For this review, take the finished solid that the model builds, in its own axes (mm). Give positions to 0.01 mm unless a question says otherwise; leave off trailing zeros. Write each loop counter-clockwise with the first axis right and the second up, starting at its lowest first coordinate (ties: lowest second). Pieces come first, ordered by that corner, then holes. Notation, with made-up numbers: M 14.5,-40 L 56.5,-40 A18 cw 56.5,-36 Z; hole C 56,-10 d2. An arc over 180 degrees is marked long. Use one line per item in the form item = value. Start each with the question number.
Q1. For probe 1 along Y at (x, z) = (2, 191); probe 2 along X at (y, z) = (-0.5, -171.5), list the stretches that pass through material, from the lowest coordinate up. Write a range as [from, to].
Q2. Clearance check with flat-ended pins moving along their axes: pin 1 Ø8 at (x, z) = (4.5, -220) entering from +Y; pin 2 Ø2 at (x, z) = (-11.5, -84.5) entering from +Y; pin 3 Ø10 at (x, y) = (11.5, -2) entering from +Z. State where each tip first meets the part, or that it passes through.
Q3. Consider section A-A on z = 134. Write out the cut boundary in (x, y).
```python
from build123d import *

# Parameters (mm, degrees)
SKETCH1_R           = 20
BOSS_EXTRUDE1_DEPTH = 262.5
FILLET1_R           = 10


with BuildPart() as part:
    # Sketch1 → Boss-Extrude1 (new body, symmetric)
    with BuildSketch(Plane.XY):
        Circle(SKETCH1_R)
    extrude(amount=BOSS_EXTRUDE1_DEPTH, both=True)

    # Sketch2 → Revolve1 (revolve)
    with BuildSketch(Plane(origin=(0, 0, 0), x_dir=(0, 0, -1), z_dir=(1, 0, 0))):
        with BuildLine():
            Line((-262.5, 20), (-262.5, 0))
            Line((-262.5, 0), (-282.5, 0))
            ThreePointArc((-282.5, 0), (-279.57043003, 9.686707526), (-271.763715382, 16.126419422))
            Line((-271.763715382, 16.126419422), (-262.5, 20))
        make_face()
    revolve1 = revolve(axis=Axis((0, 0, 262.5), (0, 0, 1)))

    # Mirror1: Revolve1 across plane
    add(revolve1.mirror(Plane.XY))

    # Fillet1
    fillet1_edges = [part.edges().sort_by_distance(p)[0] for p in [
        (14.142135624, 14.142135624, 262.5),
        (-14.142135624, -14.142135624, -262.5),
    ]]
    fillet(fillet1_edges, radius=FILLET1_R)


solid = part.part
```
Working result:
q1.probe_1 = [-19.9, 19.9]
q1.probe_2 = [-19.99, 19.99]
q2.pin_1 = 19.99
q2.pin_2 = 17.02
q2.pin_3 = 281.18
q3.outline = C 0,0 d40
